```python
from build123d import *

# Parameters (mm, degrees)
EXTRUDE_THIN1_DEPTH = 31
FILLET1_R           = 8


with BuildPart() as part:
    # Sketch1 → Extrude-Thin1 (new, symmetric)
    with BuildSketch(Plane(origin=(0, 0, 0), x_dir=(1, 0, 0), z_dir=(0, 1, 0))):
        with BuildLine():
            Line((152.47855459256846, -515.8635684817917), (152.7896920748552, -507.8696211797939))
            Line((152.7896920748552, -507.8696211797939), (158.5314712170514, -360.34808328894457))
            ThreePointArc((158.5314712170514, -360.3480832889447), (137.27301850763482, -323.2785971562588), (94.64239044734069, -326.2278623062159))
            Line((94.64239044734076, -326.22786230621585), (-35.939394152340476, -421.1695886755354))
            Line((-35.939394152340476, -421.1695886755354), (-26.236355613015643, -434.5150389528538))
            Line((-26.236355613015643, -434.5150389528538), (104.3454289866656, -339.57331258353423))
            ThreePointArc((104.34542898666567, -339.5733125835342), (129.50014740733602, -337.8330629608887), (142.04395490668114, -359.70636223172806))
            Line((142.04395490668114, -359.7063622317282), (136.30217576448493, -507.2279001225775))
            Line((136.30217576448493, -507.2279001225775), (135.9910382821982, -515.2218474245752))
            Line((135.9910382821982, -515.2218474245752), (152.47855459256846, -515.8635684817917))
        make_face()
    extrude(amount=EXTRUDE_THIN1_DEPTH, both=True)

    # Fillet1
    fillet1_edges = [part.edges().sort_by_distance(p)[0] for p in [
        (152.47855459256846, 0, 515.8635684817917),
        (135.9910382821982, 0, 515.2218474245752),
        (-26.236355613015643, 0, 434.5150389528538),
        (-35.939394152340476, 0, 421.1695886755354),
    ]]
    fillet(fillet1_edges, radius=FILLET1_R)


solid = part.part
```
Model file for the job. Use its own axes, mm. A direction names the side the tool comes from. Give positions to 0.01 mm unless a question says otherwise; leave off trailing zeros. Loops run counter-clockwise (first coordinate to the right, second up) from the corner with the lowest first, then second, coordinate; pieces in that order, holes last. Notation, with made-up numbers: (28.5, 20.25) -> (46.5, 20.25) arc R34 cw to (46.5, 53.25) -> close; hole circle Ø6 at (70.25, 5). An arc over 180 degrees is marked (long way). Write each question's results on one line, items separated by ' | '.
(1) Flat gauge pins, fed straight in: pin 1 Ø1 at (y, z) = (12.5, 376.5) entering from -X; pin 2 Ø4 at (y, z) = (-7.5, 492.5) entering from +X; pin 3 Ø2 at (y, z) = (14, 469.5) entering from +X. Where does each tip first touch, or does it go through?
Geometry results:
pin 1: stops at x = 24.81 | pin 2: stops at x = 153.47 | pin 3: stops at x = 154.32
(2) Cut at D-D on x = 40.5. List the corners of the cut face in (y, z).
Geometry results:
outline: (-31, 365.59) -> (31, 365.59) -> (31, 385.99) -> (-31, 385.99) -> close
(3) Cut at A-A on y = 13.5. List the corners of the cut face in (x, z).
Geometry results:
outline: (-31.23, 427.64) arc R8 ccw to (-29.47, 416.47) -> (94.64, 326.23) arc R40.25 ccw to (158.53, 360.35) -> (152.79, 507.87) arc R8 ccw to (144.48, 515.55) -> (143.98, 515.53) arc R8 ccw to (136.3, 507.23) -> (142.04, 359.71) arc R23.75 cw to (104.35, 339.57) -> (-19.77, 429.81) arc R8 ccw to (-30.94, 428.04) -> close
(4) Cut at B-B on z = 425. List the corners of the cut face in (x, y), and give its area (3 significant figures).
Geometry results:
outline: (-32.49, -31) -> (-13.15, -31) -> (-13.15, 31) -> (-32.49, 31) -> close; (139.5, -31) -> (156.02, -31) -> (156.02, 31) -> (139.5, 31) -> close | area: 2,220 mm²
(5) Tool access for faces 1 (the cylindrical face through (129.17, 0.43, 337.66)), 2 (the flat face through (140.4, 31, 409.3)), 3 (the flat face through (41.421, 0.434, 385.324)): list every direction of +Z, -Z, +X, -X, +Y, -Y with a clear straight run to the whole face (end or side of a thin tool).
Geometry results:
face 1: +Y, -Y | face 2: +Z, -Z, +X, -X, +Y | face 3: +Z, +Y, -Y
(6) Cut at C-C on z = 382.5. List the corners of the cut face in (x, y).
Geometry results:
outline: (17.25, -31) -> (45.3, -31) -> (45.3, 31) -> (17.25, 31) -> close; (141.16, -31) -> (157.67, -31) -> (157.67, 31) -> (141.16, 31) -> close
(7) Probe line 1 along X through (y, z) = (25, 360); line 2 along X through (y, z) = (-12.5, 391); line 3 along Z through (x, y) = (28.5, 2). List the from-to ranges inside material, lowest first.
Geometry results:
line 1: x = 48.19 to 76.25, 142.03 to 158.54 | line 2: x = 5.56 to 33.61, 140.83 to 157.34 | line 3: z = 374.32 to 394.72
